Input: part model. Units: mm. Frame: model coordinates. Face numbers are marked on the shaded views. A direction names the side the tool comes from. Give positions to 0.01 mm unless a question says otherwise; leave off trailing zeros. Loops run counter-clockwise (first coordinate to the right, second up) from the corner with the lowest first, then second, coordinate; pieces in that order, holes last. Notation, with made-up numbers: (-27.75, 83.5) -> (14.25, 83.5) arc R25 ccw to (14.25, 121.5) -> close; hole circle Ø10 at (-22.75, 85.25). An arc over 180 degrees is marked (long way). Use CSV: the item, a comma, the result in double quotes.
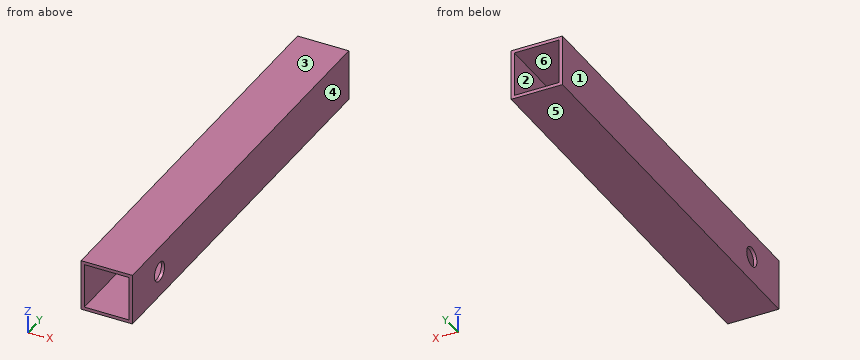
Autodesk Inventor part; units mm, degrees
ref_plane "YZ Plane" through (0, 0, 0) normal (1, 0, 0) x (0, 1, 0)
ref_plane "XZ Plane" through (0, 0, 0) normal (0, 1, 0) x (-1, 0, 0)
ref_plane "XY Plane" through (0, 0, 0) normal (0, 0, 1) x (1, 0, 0)
sketch "Sketch1" plane through (0, 0, 0) normal (0, 0, 1) x (1, 0, 0)
  line L0 (0, 0) -> (25.4, 0)
  line L1 (25.4, 0) -> (25.4, 203.2)
  line L2 (25.4, 203.2) -> (0, 203.2)
  line L3 (0, 203.2) -> (0, 0)
  dimension "d0" = 203.2
  dimension "d1" = 25.4
extrude "Extrusion1" add sketch "Sketch1" along normal blind 25.4
shell "Shell1" thickness 1.5875 removed faces 2 at (16.9333, 203.2, 8.4667) at (8.4667, 0, 8.4667)
sketch "Sketch2" plane through (25.4, 0, 0) normal (1, 0, 0) x (0, 0, -1)
  line L0 (-25.4, 203.2) -> (-25.4, 0)
  line L1 (0, 0) -> (-25.4, 0)
  circle A0 centre (-12.7, 25.4) radius 4.7625
  dimension "d5" = 25.4
  dimension "d6" = 12.7
  dimension "d7" = 9.525
extrude "Extrusion2" cut sketch "Sketch2" against normal through all
properties part number "VerticalConveyorSupport" material "Aluminum-6061"
1) Section query C-C (x = 20). Return loops of the section in (y, z), then the cut area to 3 significant figures.
From the geometry:
outline,"(0, 0) -> (203.2, 0) -> (203.2, 1.59) -> (0, 1.59) -> close; (0, 23.81) -> (203.2, 23.81) -> (203.2, 25.4) -> (0, 25.4) -> close"
area,"645 mm^2"
2) Reachability of the marked faces 1 and 2 from +Z, -Z, +X, -X, +Y, -Y: full face, straight path, thin tool, end or side. Return the list, or none.
From the geometry:
face 1,"+Z, -Z, -X, +Y, -Y"
face 2,"+Y, -Y"
3) Section query D-D (y = 25.4). Return loops of the section in (x, z), then the cut area to 3 significant figures.
From the geometry:
outline,"(0, 0) -> (25.4, 0) -> (25.4, 7.94) -> (23.81, 7.94) -> (23.81, 1.59) -> (1.59, 1.59) -> (1.59, 7.94) -> (0, 7.94) -> close; (0, 17.46) -> (1.59, 17.46) -> (1.59, 23.81) -> (23.81, 23.81) -> (23.81, 17.46) -> (25.4, 17.46) -> (25.4, 25.4) -> (0, 25.4) -> close"
area,"121 mm^2"
4) Contact query for flat-ended pins moving along their axis: pin 1 (2 mm diameter, centred on y = 38, z = 17.5, fed in from -X); pin 2 (6 mm diameter, centred on x = 6.5, z = 5.5, fed in from +Y). Output: stop coordinate, or through.
From the geometry:
pin 1,"stops at x = 0"
pin 2,"passes through"
5) Ray query, line 1 (Z direction, x = 16.5, y = 37.5); line 2 (Y direction, x = 0.65, z = 12.7). Return the intervals inside material, ascending.
From the geometry:
line 1,"z = 0 to 1.59, 23.81 to 25.4"
line 2,"y = 0 to 20.64, 30.16 to 203.2"
6) Mould query, pull axis Z, two halves, no side actions, for the marked faces 3, 4, 5 and 6. Classes: pulls with the +Z half, pulls with the -Z half, needs draft (parallel to the pull), parting line crosses it, or undercut.
From the geometry:
face 3,"pulls with the +Z half"
face 4,"needs draft"
face 5,"pulls with the -Z half"
face 6,"undercut"
7) Section query B-B (y = 51). Return loops of the section in (x, z), then the cut area to 3 significant figures.
From the geometry:
outline,"(0, 0) -> (25.4, 0) -> (25.4, 25.4) -> (0, 25.4) -> close; hole (1.59, 1.59) -> (23.81, 1.59) -> (23.81, 23.81) -> (1.59, 23.81) -> close"
area,"151 mm^2"
8) Section query A-A (z = 12.7). Return loops of the section in (x, y), then the cut area to 3 significant figures.
From the geometry:
outline,"(0, 0) -> (1.59, 0) -> (1.59, 20.64) -> (0, 20.64) -> close; (0, 30.16) -> (1.59, 30.16) -> (1.59, 203.2) -> (0, 203.2) -> close; (23.81, 0) -> (25.4, 0) -> (25.4, 20.64) -> (23.81, 20.64) -> close; (23.81, 30.16) -> (25.4, 30.16) -> (25.4, 203.2) -> (23.81, 203.2) -> close"
area,"615 mm^2"
